Autodesk Inventor part; units mm, degrees
ref_plane "YZ Plane" through (0, 0, 0) normal (1, 0, 0) x (0, 1, 0)
ref_plane "XZ Plane" through (0, 0, 0) normal (0, 1, 0) x (-1, 0, 0)
ref_plane "XY Plane" through (0, 0, 0) normal (0, 0, 1) x (1, 0, 0)
sketch "Sketch1" plane through (0, 0, 0) normal (0, 0, 1) x (1, 0, 0)
  point P0 (0, 0)
sketch "Sketch2" plane through (0, 0, 0) normal (0, 0, 1) x (1, 0, 0)
  line L0 (-100, -34.5) -> (-100, 34.5)
  circle A0 centre (-60, 22) radius 1.4998
  circle A1 centre (-60, -22) radius 1.4998
  circle A2 centre (-89.5, 25) radius 14.1598
  circle A3 centre (-89.5, -25) radius 14.1598
  line L1 (-32, 34.5) -> (-32, -34.5)
  line L2 (-32, 34.5) -> (-100, 34.5)
  line L3 (-32, -34.5) -> (-100, -34.5)
  circle A4 centre (-90.5, 25.5) radius 1.5
  circle A5 centre (-90.5, -25.5) radius 1.5
  circle A6 centre (-39.5, 25.5) radius 1.5
  circle A7 centre (-39.5, -25.5) radius 1.5
  point P0 (-100, 15.5)
  point P1 (-100, -15.5)
  point P2 (-79, -34.5)
  point P3 (-79, 34.5)
extrude "Extrusion1" add sketch "Sketch2" along normal blind 3 contours A3 L0 | L3 A3 | L0 A3 L3 | L0 A2 L2 L1 L3 A3 | A2 L0 | L0 L2 A2 | A2 L2 | A4 | A5 | A6 | A7
fillet "Fillet2" radius 4 2 edges at (-32, 34.5, 1.5) (-32, -34.5, 1.5)
extrude "Extrusion2" cut sketch "Sketch2" along normal blind 10 contours A4 | A5 | A6 | A7
properties part number "Power Distribution Board redo v2" material "CFRP"
Here's how the part is built. I have some questions about the finished solid (model axes, mm). A direction names the side the tool comes from. Give positions to 0.01 mm unless a question says otherwise; leave off trailing zeros. Write each loop counter-clockwise with the first axis right and the second up, starting at its lowest first coordinate (ties: lowest second). Pieces come first, ordered by that corner, then holes. Notation, with made-up numbers: (29, 88) -> (54, 88) arc R25 cw to (54, 126) -> close; hole circle Ø7 at (3.5, 70.5). An arc over 180 degrees is marked (long way). Use one line per item in the form item = value.
1) On a 3-axis mill with a long thin cutter (end or side, diameter ignored), from which of +Z, -Z, +X, -X, +Y, -Y can I reach the whole of each face in a straight line? I mean faces 4 (the face through (-100, 0, 1)), 5 (the face through (-32, 0, 1)), 6 (the face through (-57, 34.5, 1)), 7 (the face through (-57, -34.5, 1)). Say none if no direction works.
Verdict:
face_4 = +Z, -Z, -X
face_5 = +Z, -Z, +X, +Y, -Y
face_6 = +Z, -Z, +X, +Y
face_7 = +Z, -Z, +X, -Y
2) Suppose I cut it at B-B (x = -39.5). Please give me the cut outline in (y, z).
Verdict:
outline = (-34.5, 0) -> (-27, 0) -> (-27, 3) -> (-34.5, 3) -> close; (-24, 0) -> (24, 0) -> (24, 3) -> (-24, 3) -> close; (27, 0) -> (34.5, 0) -> (34.5, 3) -> (27, 3) -> close
3) I'm going to push flat-ended pins straight in: pin 1 (1 mm diameter, centred on y = -26.5, z = 1.5, fed in from -X); pin 2 (1.5 mm diameter, centred on x = -59.5, z = 1.5, fed in from -Y). Where does each tip first touch, or does it pass through?
Verdict:
pin_1 = -103.62
pin_2 = -34.5
4) Suppose I cut it at C-C (y = -25.5). Please give me the cut outline in (x, z), and give its area (3 significant figures).
Verdict:
outline = (-103.65, 0) -> (-92, 0) -> (-92, 3) -> (-103.65, 3) -> close; (-89, 0) -> (-41, 0) -> (-41, 3) -> (-89, 3) -> close; (-38, 0) -> (-32, 0) -> (-32, 3) -> (-38, 3) -> close
area = 197 mm2
5) We'd pull the mould along X, two halves only. Please class faces 1 (the face through (-98.767, -35.706, 1.479)), 2 (the face through (-58.57, 21.55, 1.48)), 3 (the face through (-33.141, 33.297, 1.521)): +X half, -X half, draft (parallel to the pull), parting line (faces both ways), or undercut.
Verdict:
face_1 = parting line
face_2 = undercut
face_3 = +X half
6) Suppose I cut it at D-D (y = 22). Please give me the cut outline in (x, z), and give its area (3 significant figures).
Verdict:
outline = (-103.34, 0) -> (-61.5, 0) -> (-61.5, 3) -> (-103.34, 3) -> close; (-58.5, 0) -> (-32, 0) -> (-32, 3) -> (-58.5, 3) -> close
area = 205 mm2
7) If I drill on L1, parallel to Y at x = -60, z = 1.6; L2, parallel to X at y = -25.5, z = 1.3; L3, parallel to Y at x = -39.5, z = 1, over which ranges is the centre line in solid material (lowest first)? Write a range as [from, to].
Verdict:
L1 = [-34.5, -23.5], [-20.5, 20.5], [23.5, 34.5]
L2 = [-103.65, -92], [-89, -41], [-38, -32]
L3 = [-34.5, -27], [-24, 24], [27, 34.5]
8) Suppose I cut it at A-A (z = 0.6). Please give me the cut outline in (x, y).
Verdict:
outline = (-100, -15.5) arc R14.16 ccw to (-79, -34.5) -> (-36, -34.5) arc R4 ccw to (-32, -30.5) -> (-32, 30.5) arc R4 ccw to (-36, 34.5) -> (-79, 34.5) arc R14.16 ccw to (-100, 15.5) -> close; hole circle Ø3 at (-90.5, -25.5); hole circle Ø3 at (-90.5, 25.5); hole circle Ø3 at (-60, -22); hole circle Ø3 at (-60, 22); hole circle Ø3 at (-39.5, -25.5); hole circle Ø3 at (-39.5, 25.5)
